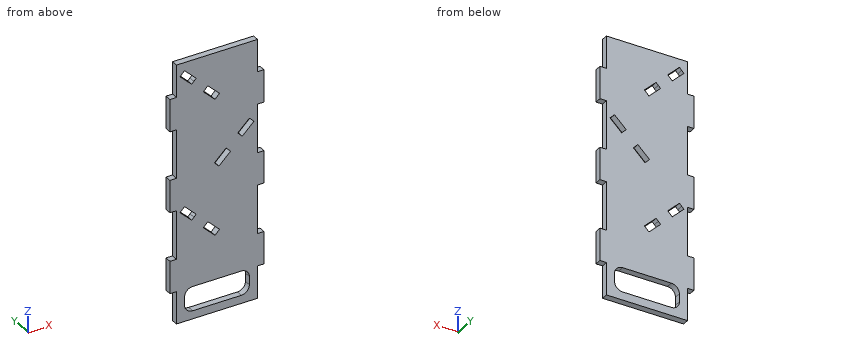
from build123d import *

# Parameters (mm, degrees)
F0_W     = 50
F0_H     = 160
F1_DEPTH = 4
F2_W     = 4
F2_H     = 20
F2_H_2   = 10
F3_DEPTH = 4
F4_W     = 40
F4_H     = 15
F5_DEPTH = 25
F6_R     = 5


with BuildPart() as f1:
    # F0 (on Front) → F1 (new body)
    with BuildSketch(Plane.XZ):
        Rectangle(F0_W, F0_H)
        Polygon((-21.403301, -10.473292), (-20.013984, -9.034612), (-12.820586, -15.981196), (-14.209903, -17.419876), (-15.59922, -18.858555), (-22.792618, -11.911971), align=None, mode=Mode.SUBTRACT)
        Polygon((-1.212424, -32.751723), (-8.405822, -25.805139), (-7.016505, -24.366459), (-5.627188, -22.92778), (1.56621, -29.874363), (0.176893, -31.313043), align=None, mode=Mode.SUBTRACT)
        Polygon((-22.792618, 72.088029), (-21.403301, 73.526708), (-20.013984, 74.965388), (-12.820586, 68.018804), (-14.209903, 66.580124), (-15.59922, 65.141445), align=None, mode=Mode.SUBTRACT)
        Polygon((-8.405822, 58.194861), (-7.016505, 59.633541), (-5.627188, 61.07222), (1.56621, 54.125637), (0.176893, 52.686957), (-1.212424, 51.248277), align=None, mode=Mode.SUBTRACT)
        Polygon((5.627188, 19.07222), (7.016505, 17.633541), (8.405822, 16.194861), (1.212424, 9.248277), (-0.176893, 10.686957), (-1.56621, 12.125637), align=None, mode=Mode.SUBTRACT)
        Polygon((20.013984, 32.965388), (21.403301, 31.526708), (22.792618, 30.088029), (15.59922, 23.141445), (14.209903, 24.580124), (12.820586, 26.018804), align=None, mode=Mode.SUBTRACT)
    extrude(amount=F1_DEPTH)

    # F2 (on face) → F3 (join)
    with BuildSketch(Plane.XZ.offset(4)):
        with Locations((-27, 50)):
            Rectangle(F2_W, F2_H)
        with Locations((-27, -5)):
            Rectangle(F2_W, F2_H_2)
        with Locations((-27, 5)):
            Rectangle(F2_W, F2_H_2)
        with Locations((-27, -50)):
            Rectangle(F2_W, F2_H)
        with Locations((27, 5)):
            Rectangle(F2_W, F2_H_2)
        with Locations((27, -5)):
            Rectangle(F2_W, F2_H_2)
        with Locations((27, 50)):
            Rectangle(F2_W, F2_H)
        with Locations((27, -50)):
            Rectangle(F2_W, F2_H)
    extrude(amount=-F3_DEPTH)

    # F4 (on face) → F5 (cut)
    with BuildSketch(Plane.XZ.offset(4)):
        with Locations((0, -67.5)):
            Rectangle(F4_W, F4_H)
    extrude(amount=-F5_DEPTH, mode=Mode.SUBTRACT)

    # F6
    f6_edges = [f1.edges().sort_by_distance(p)[0] for p in [
        (-20, -2, -60),
        (20, -2, -60),
        (20, -2, -75),
        (-20, -2, -75),
    ]]
    fillet(f6_edges, radius=F6_R)


solid = f1.part
Work out the finished part from the listing and answer in its coordinate system (mm). Give positions to 0.01 mm unless a question says otherwise; leave off trailing zeros. Order: outer loops, then holes, each group sorted by start corner. A loop starts at its lowest first (then second) coordinate and runs counter-clockwise, first axis right, second up. Notation, with made-up numbers: (12.25, 8) -> (54.25, 8) arc R23 cw to (54.25, 39) -> close; hole circle Ø2 at (61, 70.25). An arc over 180 degrees is marked (long way). Answer as a JSON object with one key per item and string values. Group by question number.
1. Section B-B on y = -3.35 is taken. Count the separate pieces of the cut face and the enclosed holes in it, plus the area to 3 significant figures.
2. Section A-A on x = -3.5 is taken. Determine the outline of the cut face in (y, z), plus the area to 3 significant figures.
3. Flat-ended cylindrical pins translate along their axes: pin 1 Ø1.2 at (y, z) = (-3, -23.5) entering from +X; pin 2 Ø1.2 at (x, y) = (27.5, -2) entering from +Z; pin 3 Ø1.2 at (y, z) = (-1, 23) entering from -X. Find the tip coordinate at first contact, or state that the pin passes through.
4. Consider line 1 along Z through (x, y) = (-25.5, -0.7); line 2 along Z through (x, y) = (-21.5, -3.25); line 3 along Z through (x, y) = (-19, -1.8). Determine where each line is inside the solid, lowest interval first. Write a range as [from, to].
Result sheet:
{
 "1": {"separate pieces": "1", "enclosed holes": "7", "area": "7,660 mm^2"},
 "2": {"outline": "(-4, -80) -> (0, -80) -> (0, -75) -> (-4, -75) -> close; (-4, -60) -> (0, -60) -> (0, -30.54) -> (-4, -30.54) -> close; (-4, -24.98) -> (0, -24.98) -> (0, 53.46) -> (-4, 53.46) -> close; (-4, 59.02) -> (0, 59.02) -> (0, 80) -> (-4, 80) -> close", "area": "536 mm^2"},
 "3": {"pin 1": "stops at x = 25", "pin 2": "stops at z = 60", "pin 3": "stops at x = -25"},
 "4": {"line 1": "z = [-60, -40], [-10, 10], [40, 60]", "line 2": "z = [-80, -13.16], [-10.57, 70.84], [73.43, 80]", "line 3": "z = [-80, -73], [-62, -15.57], [-10.01, 68.43], [73.99, 80]"}
}
